Read the model definition and answer for the solid it produces. Units are mm, in the model's axes. A direction names the side the tool comes from. Give positions to 0.01 mm unless a question says otherwise; leave off trailing zeros. Order: outer loops, then holes, each group sorted by start corner. A loop starts at its lowest first (then second) coordinate and runs counter-clockwise, first axis right, second up. Notation, with made-up numbers: (46.5, 15.25) -> (93.5, 15.25) arc R26 cw to (93.5, 32.25) -> close; hole circle Ø8 at (-13.5, 15). An arc over 180 degrees is marked (long way). Answer as CSV lines item,"result". Start each with the question number.
1) Flat-ended cylindrical pins translate along their axes: pin 1 Ø2 at (y, z) = (1, 7) entering from -X; pin 2 Ø1.2 at (x, z) = (26, 1.5) entering from +Y; pin 3 Ø3 at (x, y) = (24, 5) entering from +Z; pin 4 Ø4.5 at (x, z) = (24, 2.5) entering from -Y. Find the tip coordinate at first contact, or state that the pin passes through.
2) For faces 1 (the face through (5, 5, 1)), 2 (the face through (24, 7, 2)), 3 (the face through (24, 5, 4)), 4 (the face through (24, 3, 2)), determine the directions among +Z, -Z, +X, -X, +Y, -Y from which every point of the face is accessible in a straight line to the end or side of a thin tool.
3) Find section C-C (y = 5). Determine the outline of the cut face in (x, z), and give its area (3 significant figures).
4) Find section B-B (z = 2.5). Determine the outline of the cut face in (x, y).
5) Find section D-D (z = 4.5). Determine the outline of the cut face in (x, y), and give its area (3 significant figures).
6) Straight lines are drawn through the part: L1, parallel to Z at x = 3.5, y = 5.5; L2, parallel to Y at x = 7.25, z = 3; L3, parallel to X at y = 4.25, z = 6.5. For each, find the intervals that lie inside material, in ascending order. Write a range as from..to.
7) The mould has two halves that part along Y. Classify faces 5 (the face through (5, 2.25, 3)), 6 (the face through (5, 5, 6)), 7 (the face through (10, 0, 5)), 8 (the face through (20, 5, 5)): +Y half, -Y half, draft (parallel to the pull), parting line (faces both ways), or undercut.
8) Find section A-A (x = 3.75). Determine the outline of the cut face in (y, z).
```python
from build123d import *

# Parameters (mm, degrees)
F0_W     = 20
F0_H     = 10
F1_DEPTH = 10
F2_W     = 4
F2_H     = 4
F3_DEPTH = 9
F4_W     = 5.5
F4_H     = 5
F5_DEPTH = 10


with BuildPart() as f1:
    # F0 (on Top) → F1 (new body)
    with BuildSketch(Plane.XY):
        with Locations((10, 5)):
            Rectangle(F0_W, F0_H)
    extrude(amount=F1_DEPTH)

    # F2 (on face) → F3 (join)
    with BuildSketch(Plane.YZ.offset(20)):
        with Locations((5, 2)):
            Rectangle(F2_W, F2_H)
    extrude(amount=F3_DEPTH)

    # F4 (on face) → F5 (cut)
    with BuildSketch(Plane(origin=(0, 0, 0), x_dir=(0, -1, 0), z_dir=(-1, 0, 0))):
        with Locations((-5, 3.5)):
            Rectangle(F4_W, F4_H)
    extrude(amount=-F5_DEPTH, mode=Mode.SUBTRACT)


solid = f1.part
```
Findings below:
1,pin 1,"x = 0"
1,pin 2,"y = 7"
1,pin 3,"z = 4"
1,pin 4,"y = 3"
2,face 1,"-X"
2,face 2,"+Z, -Z, +X, +Y"
2,face 3,"+Z, +X, +Y, -Y"
2,face 4,"+Z, -Z, +X, -Y"
3,outline,"(0, 0) -> (29, 0) -> (29, 4) -> (20, 4) -> (20, 10) -> (0, 10) -> (0, 6) -> (10, 6) -> (10, 1) -> (0, 1) -> close"
3,area,"186 mm²"
4,outline,"(0, 0) -> (20, 0) -> (20, 3) -> (29, 3) -> (29, 7) -> (20, 7) -> (20, 10) -> (0, 10) -> (0, 7.75) -> (10, 7.75) -> (10, 2.25) -> (0, 2.25) -> close"
5,outline,"(0, 0) -> (20, 0) -> (20, 10) -> (0, 10) -> (0, 7.75) -> (10, 7.75) -> (10, 2.25) -> (0, 2.25) -> close"
5,area,"145 mm²"
6,L1,"0..1, 6..10"
6,L2,"0..2.25, 7.75..10"
6,L3,"0..20"
7,face 5,"undercut"
7,face 6,"undercut"
7,face 7,"-Y half"
7,face 8,"draft"
8,outline,"(0, 0) -> (10, 0) -> (10, 10) -> (0, 10) -> close; hole (2.25, 1) -> (7.75, 1) -> (7.75, 6) -> (2.25, 6) -> close"
